from build123d import *
from OCP.BRepFilletAPI import BRepFilletAPI_MakeChamfer

# Parameters (mm, degrees)
BOSS_EXTRUDE1_DEPTH      = 50
BOSS_EXTRUDE1_DEPTH_BACK = 150
SKETCH1_R                = 6
SKETCH2_R                = 4
BOSS_EXTRUDE2_DEPTH      = 25
SKETCH3_R                = 6
BOSS_EXTRUDE3_DEPTH      = 8
CHAMFER1_SIZE            = 2
CHAMFER1_SIZE2           = 1.154700538
CHAMFER2_SIZE            = 2
FILLET1_R                = 0.5


with BuildPart() as part:
    # Sketch1 → Boss-Extrude1 (new, two sides: drawn at the far end of the back side and taken through both)
    with BuildSketch(Plane.XY.offset(-BOSS_EXTRUDE1_DEPTH_BACK)):
        Circle(SKETCH1_R)
    extrude(amount=BOSS_EXTRUDE1_DEPTH + BOSS_EXTRUDE1_DEPTH_BACK)

    # Sketch2 → Boss-Extrude2 (add)
    with BuildSketch(Plane(origin=(0, 0, 0), x_dir=(1, 0, 0), z_dir=(0, 1, 0))):
        with Locations(Location((0, -30, 0), (0, 0, 90))):
            Circle(SKETCH2_R)
    extrude(amount=BOSS_EXTRUDE2_DEPTH)

    # Sketch3 → Boss-Extrude3 (add)
    with BuildSketch(Plane(origin=(0, 25, 0), x_dir=(1, 0, 0), z_dir=(0, 1, 0))):
        with Locations(Location((0, -30, 0), (0, 0, 270))):
            Circle(SKETCH3_R)
    extrude(amount=-BOSS_EXTRUDE3_DEPTH)

    # Chamfer1: one chamfer whose edges measure the first distance from different faces: ONE call of the kernel's chamfer builder (chamfer() names one face for all edges)
    chamfer1_edges_1 = [part.edges().sort_by_distance(p)[0] for p in [
        (-6, 0, 50),
    ]]
    chamfer1_side_1 = [part.faces().sort_by_distance(p)[0] for p in [
        (-6, 0, 25),
    ]]
    chamfer1_edges_2 = [part.edges().sort_by_distance(p)[0] for p in [
        (-6, 0, -150),
    ]]
    chamfer1_side_2 = [part.faces().sort_by_distance(p)[0] for p in [
        (-6, 0, -75),
    ]]
    chamfer1 = BRepFilletAPI_MakeChamfer(part.part.solid().wrapped)
    for e in chamfer1_edges_1:
        chamfer1.Add(CHAMFER1_SIZE, CHAMFER1_SIZE2, e.wrapped, chamfer1_side_1[0].wrapped)  # the first distance lies on this face
    for e in chamfer1_edges_2:
        chamfer1.Add(CHAMFER1_SIZE, CHAMFER1_SIZE2, e.wrapped, chamfer1_side_2[0].wrapped)  # the first distance lies on this face
    add(Compound.cast(chamfer1.Shape()), mode=Mode.REPLACE)

    # Chamfer2
    chamfer2_edges = [part.edges().sort_by_distance(p)[0] for p in [
        (0, 17, 24),
    ]]
    chamfer(chamfer2_edges, length=CHAMFER2_SIZE - 0.0001)  # a hair under: the kernel refuses the full size

    # Fillet1
    fillet1_edges = [part.edges().sort_by_distance(p)[0] for p in [
        (0, 18.9999, 24),
        (0, 25, 24),
    ]]
    fillet(fillet1_edges, radius=FILLET1_R)


solid = part.part
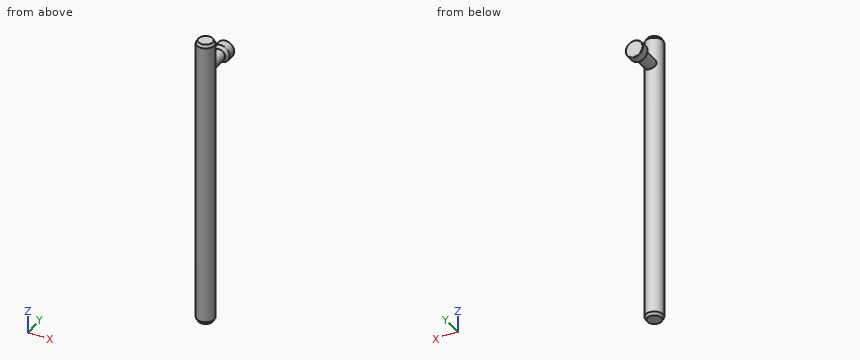
Input: part model. Units: mm. Frame: model coordinates. Give positions to 0.01 mm unless a question says otherwise; leave off trailing zeros. Write each loop counter-clockwise with the first axis right and the second up, starting at its lowest first coordinate (ties: lowest second). Pieces come first, ordered by that corner, then holes. Notation, with made-up numbers: M 79.25,78 L 110.25,78 A29 cw 110.25,114 Z; hole C 4.5,64.25 d8. An arc over 180 degrees is marked long. Write item = value, one per line. Start each with the question number.
1) First-contact query: pin 1 Ø1 at (x, z) = (-2.5, -98.5) entering from +Y; pin 2 Ø1.5 at (x, y) = (1.5, 9) entering from -Z; pin 3 Ø3 at (y, z) = (3.5, 25.5) entering from +X; pin 4 Ø3 at (y, z) = (9, -59.5) entering from -X. Flat tips, straight axial feed; report the tip coordinate or a pass-through.
2) Cut plane B-B on y = 22.5. Return the cut outline in (x, z).
3) Material intervals for line 1 along Y through (x, z) = (-1.25, -82.5); line 2 along Y through (x, z) = (0.5, -121.5); line 3 along Z through (x, y) = (0.25, 23), sorted ascending. Write a range as [from, to].
4) Cut plane A-A on z = -105. Return the cut outline in (x, y), then the cut area to 3 significant figures.
Solved:
q1.pin_1 = 5.66
q1.pin_2 = 26.07
q1.pin_3 = 5.66
q1.pin_4 = through
q2.outline = C 0,30 d12
q3.line_1 = [-5.87, 5.87]
q3.line_2 = [-5.98, 5.98]
q3.line_3 = [24.01, 35.99]
q4.outline = C 0,0 d12
q4.area = 113 mm2
